Study the drawing (mm; zero at the part's minimum x, y, z) and answer. A direction names the side the tool comes from. Round coordinates to 2 decimals unless told otherwise and drop trailing zeros. Order: outer loops, then holes, each group sorted by start corner. A loop starts at its lowest first (then second) coordinate and runs counter-clockwise, first axis right, second up. Notation, with made-up numbers: (8.5, -2) - (21.5, -2) arc R9 ccw to (21.5, 10) - close; hole circle Ø4 at (-36, 28). An arc over 180 degrees is marked (long way). Put each result on its own line as item: value. Start each with the question number.
Q1. Each of these flat-tipped pins is pushed along its axis until it touches: pin 1 Ø5 at (x, y) = (18.5, 66) entering from -Z; pin 2 Ø2.5 at (x, y) = (20, 65) entering from +Z; pin 3 Ø12 at (x, z) = (17.5, 18) entering from -Y; pin 4 Ø4 at (x, y) = (115, 70) entering from +Z. Where does it stop, or does it pass through?
Q2. Section C-C on z = 16.75 is taken. Give the vertices of the cut face in (x, y).
Q3. Find the intervals of material crossed by line 1 along Y through (x, z) = (155, 2.95); line 2 along X through (y, z) = (10, 3.85); line 3 along X through (y, z) = (70, 3.25), in increasing order. Write a range as from..to.
Q4. Section A-A on z = 26.75 is taken. Give the vertices of the cut face in (x, y), then the cut area to 3 significant figures.
Q5. Section B-B on x = 34 is taken. Give the vertices of the cut face in (y, z).
Q6. Which of the six approach directions +Z, -Z, +X, -X, +Y, -Y give full straight-line access (tool end or side, diameter ignored) to the marked faces 1 and 2?
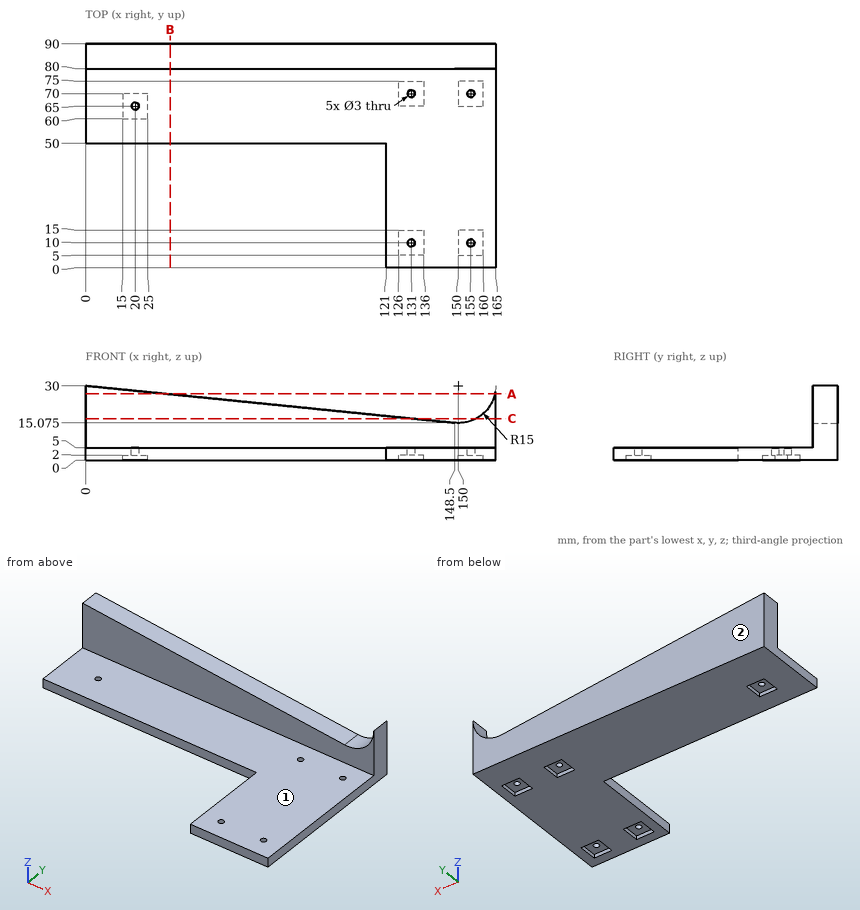
Findings:
1. pin 1: z = 2
1. pin 2: through
1. pin 3: y = 80
1. pin 4: z = 5
2. outline: (0, 80) - (131.84, 80) - (131.84, 90) - (0, 90) - close; (157.03, 80) - (165, 80) - (165, 90) - (157.03, 90) - close
3. line 1: 0..8.5, 11.5..68.5, 71.5..90
3. line 2: 121..129.5, 132.5..153.5, 156.5..165
3. line 3: 0..129.5, 132.5..153.5, 156.5..165
4. outline: (0, 80) - (32.34, 80) - (32.34, 90) - (0, 90) - close; (164.64, 80) - (165, 80) - (165, 90) - (164.64, 90) - close
4. area: 327 mm2
5. outline: (50, 0) - (90, 0) - (90, 26.58) - (80, 26.58) - (80, 5) - (50, 5) - close
6. face 1: +Z, +X, -X, -Y
6. face 2: +Z, -Z, +X, -X, +Y
